The model under review builds one solid part; all positions refer to its coordinate system, in mm. A direction names the side the tool comes from. Round coordinates to 2 decimals unless told otherwise and drop trailing zeros. Write each loop counter-clockwise with the first axis right and the second up, starting at its lowest first coordinate (ties: lowest second). Pieces come first, ordered by that corner, then holes. Notation, with made-up numbers: (78.25, 25) -> (105.25, 25) arc R25 ccw to (105.25, 59) -> close; hole circle Ø8 at (4, 87). An arc over 180 degrees is marked (long way). Return JSON: item names as keys, results as strings. Group by question number.
1. For line 1 along Y through (x, z) = (-80, 1.85); line 2 along X through (y, z) = (12.5, 2.55); line 3 along Y through (x, z) = (78, 2.3), list the stretches that pass through material, from the lowest coordinate up. Write a range as from..to.
2. Take a section at D-D, the plane x = 80. Write out the cut boundary in (y, z).
3. Take a section at B-B, the plane x = 0. Write out the cut boundary in (y, z), then the cut area to 3 significant figures.
4. Take a section at C-C, the plane y = -50. Write out the cut boundary in (x, z).
5. Clearance check with a flat-ended pin moving along its axis: P1, Ø8, axis at x = -80, y = -50, coming from the +Z side. State where the tip first meets the part, or that it passes through.
6. Tool access review of faces 4 (the flat face through (-66, 4, 3)), 5 (the cylindrical face through (-82.21, -52.03, 2.96)): name each direction out of +Z, -Z, +X, -X, +Y, -Y from which nothing blocks a thin tool from reaching the whole face with its end or side.
7. Take a section at A-A, the plane y = 50. Write out the cut boundary in (x, z), then the cut area to 3 significant figures.
8. Mouldability with a two-part tool opening along Y and no side actions: class faces 1 (the cylindrical face through (0, -53, 3)), 2 (the flat face through (66, 4, 3)), 3 (the flat face through (90, -1, 3)) as pulls with the +Y half, pulls with the -Y half, needs draft (parallel to the pull), parting line crosses it, or undercut.
Autodesk Inventor part; units mm, degrees
ref_plane "YZ Plane" through (0, 0, 0) normal (1, 0, 0) x (0, 1, 0)
ref_plane "XZ Plane" through (0, 0, 0) normal (0, 1, 0) x (-1, 0, 0)
ref_plane "XY Plane" through (0, 0, 0) normal (0, 0, 1) x (1, 0, 0)
sketch "Sketch1" plane through (0, 0, 0) normal (0, 0, 1) x (1, 0, 0)
  line L0 (-70, 40) -> (70, 40) construction
  line L1 (70, 40) -> (70, -40) construction
  line L2 (70, -40) -> (-70, -40) construction
  line L3 (-70, -40) -> (-70, 40) construction
  line L4 (90, 60) -> (-90, 60)
  line L5 (-90, 60) -> (-90, -60)
  line L6 (-90, -60) -> (90, -60)
  line L7 (90, -60) -> (90, 60)
  circle A0 centre (80, 50) radius 3
  circle A1 centre (-80, 50) radius 3
  circle A2 centre (-80, -50) radius 3
  circle A3 centre (0, -50) radius 3
  circle A4 centre (80, -50) radius 3
  line L8 (-90, 0) -> (90, 0) construction
  line L9 (0, 60) -> (0, -60) construction
  line L10 (-71, 60) -> (-71, 4)
  line L11 (-71, 4) -> (-60, 4)
  line L12 (-60, 4) -> (-60, 60)
  line L13 (71, 60) -> (71, 4)
  line L14 (71, 4) -> (60, 4)
  line L15 (60, 4) -> (60, 60)
  circle A5 centre (-35, 50) radius 3
  circle A6 centre (35, 50) radius 3
  point P0 (0, 0)
  point P1 (0, 40)
  point P2 (70, 0)
  point P3 (-70, 0)
  point P4 (0, 0)
  dimension "d0" = 140
  dimension "d1" = 80
  dimension "d2" = 20
  dimension "d7" = 6
  dimension "d8" = 10
  dimension "d9" = 10
  dimension "d17" = 56
  dimension "d18" = 11
  dimension "d19" = 1
  dimension "d20" = 10
  dimension "d21" = 35
extrude "Extrusion3" add sketch "Sketch1" along normal blind 6 contours L7 L6 L5 L4 L10 L11 L12 L15 L14 L13
properties part number "bottom"
Output:
{
 "1": {"line 1": "y = -60..-53, -47..47, 53..60", "line 2": "x = -90..-71, -60..60, 71..90", "line 3": "y = -60..-52.24, -47.76..47.76, 52.24..60"},
 "2": {"outline": "(-60, 0) -> (-53, 0) -> (-53, 6) -> (-60, 6) -> close; (-47, 0) -> (47, 0) -> (47, 6) -> (-47, 6) -> close; (53, 0) -> (60, 0) -> (60, 6) -> (53, 6) -> close"},
 "3": {"outline": "(-60, 0) -> (-53, 0) -> (-53, 6) -> (-60, 6) -> close; (-47, 0) -> (60, 0) -> (60, 6) -> (-47, 6) -> close", "area": "684 mm^2"},
 "4": {"outline": "(-90, 0) -> (-83, 0) -> (-83, 6) -> (-90, 6) -> close; (-77, 0) -> (-3, 0) -> (-3, 6) -> (-77, 6) -> close; (3, 0) -> (77, 0) -> (77, 6) -> (3, 6) -> close; (83, 0) -> (90, 0) -> (90, 6) -> (83, 6) -> close"},
 "5": {"P1": "stops at z = 6"},
 "6": {"face 4": "+Z, -Z, +Y", "face 5": "+Z, -Z"},
 "7": {"outline": "(-90, 0) -> (-83, 0) -> (-83, 6) -> (-90, 6) -> close; (-77, 0) -> (-71, 0) -> (-71, 6) -> (-77, 6) -> close; (-60, 0) -> (-38, 0) -> (-38, 6) -> (-60, 6) -> close; (-32, 0) -> (32, 0) -> (32, 6) -> (-32, 6) -> close; (38, 0) -> (60, 0) -> (60, 6) -> (38, 6) -> close; (71, 0) -> (77, 0) -> (77, 6) -> (71, 6) -> close; (83, 0) -> (90, 0) -> (90, 6) -> (83, 6) -> close", "area": "804 mm^2"},
 "8": {"face 1": "undercut", "face 2": "pulls with the +Y half", "face 3": "needs draft"}
}
